```python
from build123d import *

# Parameters (mm, degrees)
SCHIZZO3_R                   = 1.5
ESTRUSIONE_ESTRUSIONE2_DEPTH = 27.7
TAGLIO_ESTRUSIONE1_REACH     = 56.5
TAGLIO_ESTRUSIONE2_START     = -3
TAGLIO_ESTRUSIONE2_DEPTH     = 24.7
RACCORDO1_R                  = 2
SCHIZZO6_R                   = 1.6
ESTRUSIONE_ESTRUSIONE3_DEPTH = 1.5
SCHIZZO8_R                   = 1.6
ESTRUSIONE_ESTRUSIONE4_DEPTH = 2.5
RACCORDO2_R                  = 2


with BuildPart() as part:
    # Schizzo3 → Estrusione-Estrusione2 (new body)
    with BuildSketch(Plane(origin=(0, -1.8, 0), x_dir=(1, 0, 0), z_dir=(0, 1, 0))):
        with BuildLine():
            Line((27.25, -1.6), (27.25, -8.6))
            ThreePointArc((27.25, -8.6), (26.957106781, -9.307106781), (26.25, -9.6))
            Line((26.25, -9.6), (22.777350269, -9.6))
            ThreePointArc((22.777350269, -9.6), (22.277350269, -9.733974596), (21.911324865, -10.1))
            Line((21.911324865, -10.1), (20.872094381, -11.9))
            ThreePointArc((20.872094381, -11.9), (20.506068977, -12.266025404), (20.006068977, -12.4))
            Line((20.006068977, -12.4), (-20.006068977, -12.4))
            ThreePointArc((-20.006068977, -12.4), (-20.506068977, -12.266025404), (-20.872094381, -11.9))
            Line((-20.872094381, -11.9), (-21.911324865, -10.1))
            ThreePointArc((-21.911324865, -10.1), (-22.277350269, -9.733974596), (-22.777350269, -9.6))
            Line((-22.777350269, -9.6), (-26.25, -9.6))
            ThreePointArc((-26.25, -9.6), (-26.957106781, -9.307106781), (-27.25, -8.6))
            Line((-27.25, -8.6), (-27.25, -1.6))
            Line((-27.25, -1.6), (-27.25, 1.6))
            Line((-27.25, 1.6), (-27.25, 8.6))
            ThreePointArc((-27.25, 8.6), (-26.957106781, 9.307106781), (-26.25, 9.6))
            Line((-26.25, 9.6), (-22.777350269, 9.6))
            ThreePointArc((-22.777350269, 9.6), (-22.277350269, 9.733974596), (-21.911324865, 10.1))
            Line((-21.911324865, 10.1), (-20.872094381, 11.9))
            ThreePointArc((-20.872094381, 11.9), (-20.506068977, 12.266025404), (-20.006068977, 12.4))
            Line((-20.006068977, 12.4), (20.006068977, 12.4))
            ThreePointArc((20.006068977, 12.4), (20.506068977, 12.266025404), (20.872094381, 11.9))
            Line((20.872094381, 11.9), (21.911324865, 10.1))
            ThreePointArc((21.911324865, 10.1), (22.277350269, 9.733974596), (22.777350269, 9.6))
            Line((22.777350269, 9.6), (26.25, 9.6))
            ThreePointArc((26.25, 9.6), (26.957106781, 9.307106781), (27.25, 8.6))
            Line((27.25, 8.6), (27.25, 1.6))
            Line((27.25, 1.6), (27.25, -1.6))
        make_face()
        with Locations((24.2, -5)):
            Circle(SCHIZZO3_R, mode=Mode.SUBTRACT)
        with Locations((24.2, 5)):
            Circle(SCHIZZO3_R, mode=Mode.SUBTRACT)
        with Locations((-24.2, 5)):
            Circle(SCHIZZO3_R, mode=Mode.SUBTRACT)
        with Locations((-24.2, -5)):
            Circle(SCHIZZO3_R, mode=Mode.SUBTRACT)
        with BuildLine():
            Line((-19.2, -9.9), (19.2, -9.9))
            ThreePointArc((19.2, -9.9), (19.907106781, -9.607106781), (20.2, -8.9))
            Line((20.2, -8.9), (20.2, 8.9))
            ThreePointArc((20.2, 8.9), (19.907106781, 9.607106781), (19.2, 9.9))
            Line((19.2, 9.9), (-19.2, 9.9))
            ThreePointArc((-19.2, 9.9), (-19.907106781, 9.607106781), (-20.2, 8.9))
            Line((-20.2, 8.9), (-20.2, -8.9))
            ThreePointArc((-20.2, -8.9), (-19.907106781, -9.607106781), (-19.2, -9.9))
        make_face(mode=Mode.SUBTRACT)
    extrude(amount=-ESTRUSIONE_ESTRUSIONE2_DEPTH)

    # Schizzo4 → Taglio-Estrusione1 (cut, up to next)
    with BuildSketch(Plane(origin=(27.25, 0, 0), x_dir=(0, 0, -1), z_dir=(1, 0, 0)), mode=Mode.PRIVATE) as taglio_estrusione1_sk1:
        with BuildLine():
            Line((-3.710237866, -17.5387571), (3.710237866, -17.5387571))
            ThreePointArc((3.710237866, -17.5387571), (4.417344647, -17.831650319), (4.710237866, -18.5387571))
            Line((4.710237866, -18.5387571), (4.710237866, -30.61702325))
            ThreePointArc((4.710237866, -30.61702325), (4.417344647, -31.324130031), (3.710237866, -31.61702325))
            Line((3.710237866, -31.61702325), (-3.710237866, -31.61702325))
            ThreePointArc((-3.710237866, -31.61702325), (-4.417344647, -31.324130031), (-4.710237866, -30.61702325))
            Line((-4.710237866, -30.61702325), (-4.710237866, -18.5387571))
            ThreePointArc((-4.710237866, -18.5387571), (-4.417344647, -17.831650319), (-3.710237866, -17.5387571))
        make_face()
    taglio_estrusione1_tool1 = extrude(taglio_estrusione1_sk1.sketch, amount=-TAGLIO_ESTRUSIONE1_REACH, mode=Mode.PRIVATE) & part.part
    add(taglio_estrusione1_tool1.solids().sort_by_distance((27.25, -24.57789, 0))[0], mode=Mode.SUBTRACT)

    # Schizzo5 → Taglio-Estrusione2 (cut)
    with BuildSketch(Plane(origin=(0, -1.8, 0), x_dir=(1, 0, 0), z_dir=(0, 1, 0)).offset(TAGLIO_ESTRUSIONE2_START)):
        Polygon((27.25, 8.6), (27.25, -8.6), (27.507432363, -11.370727038), (21.911324865, -11.370727038), (21.911324865, -9.6), (21.911324865, 9.6), (21.911324865, 11.665734377), (27.25, 11.503675338), align=None)
    taglio_estrusione2 = extrude(amount=-TAGLIO_ESTRUSIONE2_DEPTH, mode=Mode.SUBTRACT)

    # Specchia1: Taglio-Estrusione2 across plane
    add(taglio_estrusione2.mirror(Plane(origin=(0, 0, 0), x_dir=(0, 0, 1), z_dir=(1, 0, 0))), mode=Mode.SUBTRACT)

    # Raccordo1
    raccordo1_edges = [part.edges().sort_by_distance(p)[0] for p in [
        (21.055662433, -29.5, -4.710237866),
        (21.055662433, -29.5, 4.710237866),
    ]]
    fillet(raccordo1_edges, radius=RACCORDO1_R)

    # Schizzo6 → Estrusione-Estrusione3 (add, symmetric)
    with BuildSketch(Plane.XY):
        with BuildLine():
            Line((21.911324865, -17.5387571), (30, -17.5387571))
            ThreePointArc((30, -17.5387571), (33.535533906, -16.074291006), (35, -12.5387571))
            Line((35, -12.5387571), (35, -6.8))
            ThreePointArc((35, -6.8), (33.535533906, -3.264466094), (30, -1.8))
            Line((30, -1.8), (21.911324865, -1.8))
            Line((21.911324865, -1.8), (21.911324865, -17.5387571))
        make_face()
        with Locations((30, -9.66937855)):
            Circle(SCHIZZO6_R, mode=Mode.SUBTRACT)
    estrusione_estrusione3 = extrude(amount=ESTRUSIONE_ESTRUSIONE3_DEPTH, both=True)

    # Schizzo8 → Estrusione-Estrusione4 (add)
    with BuildSketch(Plane(origin=(0, 0, -12.4), x_dir=(-1, 0, 0), z_dir=(0, 0, -1))):
        with BuildLine():
            Line((-20.006068977, -29.5), (-1.786501868, -36.469947652))
            ThreePointArc((-1.786501868, -36.469947652), (0, -36.8), (1.786501868, -36.469947652))
            Line((1.786501868, -36.469947652), (20.006068977, -29.5))
            Line((20.006068977, -29.5), (-20.006068977, -29.5))
        make_face()
        with Locations((0, -31.8)):
            Circle(SCHIZZO8_R, mode=Mode.SUBTRACT)
    extrude(amount=-ESTRUSIONE_ESTRUSIONE4_DEPTH)

    # Specchia2: Estrusione-Estrusione3 across plane
    add(estrusione_estrusione3.mirror(Plane(origin=(0, 0, 0), x_dir=(0, 0, 1), z_dir=(1, 0, 0))))

    # Raccordo2
    raccordo2_edges = [part.edges().sort_by_distance(p)[0] for p in [
        (-21.911324865, -17.5387571, 0),
    ]]
    fillet(raccordo2_edges, radius=RACCORDO2_R)


solid = part.part
```
Work out the finished part from the listing and answer in its coordinate system (mm). A direction names the side the tool comes from. Give positions to 0.01 mm unless a question says otherwise; leave off trailing zeros. Loops run counter-clockwise (first coordinate to the right, second up) from the corner with the lowest first, then second, coordinate; pieces in that order, holes last. Notation, with made-up numbers: M -33.5,67 L -6.5,67 A26 ccw -6.5,88 Z; hole C -27.5,55 d4. An arc over 180 degrees is marked long. One line per item, written item: value. Start each with the question number.
1. Each of these flat-tipped pins is pushed along its axis until it touches: P1, Ø6.5, axis at x = 30.5, y = -13.5, coming from the +Z side; P2, Ø6, axis at x = 25.5, z = 4, coming from the -Y side; P3, Ø3.5, axis at x = -24, y = -3, coming from the -Z side. Where does it stop, or does it pass through?
2. Find section C-C (y = -31.8). Give the vertices of the cut face in (x, z).
3. Find section D-D (y = -23). Give the vertices of the cut face in (x, z), and give its area (3 significant figures).
4. Find section B-B (x = 8). Give the vertices of the cut face in (y, z), and give its area (3 significant figures).
5. Determine the mould class of faces 6 (the face through (-10.769, -33.034, -11.168)), 7 (the face through (25, -3, 9.6)), 8 (the face through (22.7, -3.28, -5.07)) for opening direction X: released by +X, released by -X, zero draft, split by the parting line, or undercut.
6. Find section A-A (x = 0). Give the vertices of the cut face in (y, z).
7. Find the intervals of material crossed by probe 1 along X at (y, z) = (-4.05, 5); probe 2 along Z at (x, y) = (24, -4); probe 3 along Z at (x, y) = (-0.5, -20.5), in increasing order.
8. Which of the six approach directions +Z, -Z, +X, -X, +Y, -Y give full straight-line access (tool end or side, diameter ignored) to faces 1 (the face through (-35, -10, 0)), 2 (the face through (11.024, -32.936, -11.168)), 3 (the face through (21, -23, 4.71)), 4 (the face through (-25, -4.8, 7)), 5 (the face through (-20.2, -15, 0))?
Reported:
1. P1: stops at z = 1.5
1. P2: stops at y = -17.54
1. P3: stops at z = -9.75
2. outline: M -13.99,-12.4 L -1.6,-12.4 L -1.6,-9.9 L -13.99,-9.9 Z; M 1.6,-12.4 L 13.99,-12.4 L 13.99,-9.9 L 1.6,-9.9 Z
3. outline: M -21.91,-10.1 L -20.87,-11.9 A1 ccw -20.01,-12.4 L 20.01,-12.4 A1 ccw 20.87,-11.9 L 21.91,-10.1 L 21.91,-4.71 L 20.2,-4.71 L 20.2,-8.9 A1 cw 19.2,-9.9 L -19.2,-9.9 A1 cw -20.2,-8.9 L -20.2,8.9 A1 cw -19.2,9.9 L 19.2,9.9 A1 cw 20.2,8.9 L 20.2,4.71 L 21.91,4.71 L 21.91,10.1 L 20.87,11.9 A1 ccw 20.01,12.4 L -20.01,12.4 A1 ccw -20.87,11.9 L -21.91,10.1 Z
3. area: 265 mm²
4. outline: M -34.09,-12.4 L -1.8,-12.4 L -1.8,-9.9 L -34.09,-9.9 Z; M -29.5,9.9 L -1.8,9.9 L -1.8,12.4 L -29.5,12.4 Z
4. area: 150 mm²
5. face 6: released by -X
5. face 7: zero draft
5. face 8: undercut
6. outline: M -36.8,-12.4 L -33.4,-12.4 L -33.4,-9.9 L -36.8,-9.9 Z; M -30.2,-12.4 L -1.8,-12.4 L -1.8,-9.9 L -30.2,-9.9 Z; M -29.5,9.9 L -1.8,9.9 L -1.8,12.4 L -29.5,12.4 Z
7. probe 1: x = -27.25 to -25.7, -22.7 to -20.2, 20.2 to 22.7, 25.7 to 27.25
7. probe 2: z = -9.6 to -6.49, -3.51 to 3.51, 6.49 to 9.6
7. probe 3: z = -12.4 to -9.9, 9.9 to 12.4
8. face 1: +Z, -Z, -X, +Y, -Y
8. face 2: +Z, -Z, +X, -Y
8. face 3: +X, -Y
8. face 4: +Z, -X, -Y
8. face 5: +Y, -Y
